from build123d import *

# Parameters (mm, degrees)
SKETCH1_R               = 2.5
BOSS_EXTRUDE1_DEPTH     = 7.5
BOSS_EXTRUDE2_DEPTH     = 20
BOSS_EXTRUDE3_DEPTH     = 7
CUT_EXTRUDE_THIN1_DEPTH = 7
SKETCH5_W               = 5.5
SKETCH5_H               = 11
CUT_EXTRUDE2_DEPTH      = 4
SKETCH6_W               = 5.5
SKETCH6_H               = 11
CUT_EXTRUDE3_DEPTH      = 4


with BuildPart() as part:
    # Sketch1 → Boss-Extrude1 (new body)
    with BuildSketch(Plane(origin=(0, 0, 0), x_dir=(1, 0, 0), z_dir=(0, 1, 0))):
        with BuildLine():
            Line((33, 16.75), (42.918528102, 1.646786754))
            ThreePointArc((42.918528102, 1.646786754), (43.410920998, 0), (42.918528102, -1.646786754))
            Line((42.918528102, -1.646786754), (33, -16.75))
            Line((33, -16.75), (33, -23.75))
            ThreePointArc((33, -23.75), (32.121320344, -25.871320344), (30, -26.75))
            Line((30, -26.75), (-30, -26.75))
            ThreePointArc((-30, -26.75), (-32.121320344, -25.871320344), (-33, -23.75))
            Line((-33, -23.75), (-33, -16.75))
            Line((-33, -16.75), (-42.918528102, -1.646786754))
            ThreePointArc((-42.918528102, -1.646786754), (-43.410920998, 0), (-42.918528102, 1.646786754))
            Line((-42.918528102, 1.646786754), (-33, 16.75))
            Line((-33, 16.75), (-33, 23.75))
            ThreePointArc((-33, 23.75), (-32.121320344, 25.871320344), (-30, 26.75))
            Line((-30, 26.75), (30, 26.75))
            ThreePointArc((30, 26.75), (32.121320344, 25.871320344), (33, 23.75))
            Line((33, 23.75), (33, 16.75))
        make_face()
        with Locations((38.5, 0)):
            Circle(SKETCH1_R, mode=Mode.SUBTRACT)
        with Locations((-38.5, 0)):
            Circle(SKETCH1_R, mode=Mode.SUBTRACT)
    extrude(amount=BOSS_EXTRUDE1_DEPTH)

    # Sketch2 → Boss-Extrude2 (add)
    with BuildSketch(Plane(origin=(0, 7.5, 0), x_dir=(1, 0, 0), z_dir=(0, 1, 0))):
        with BuildLine():
            Line((-30, 18.5), (30, 18.5))
            ThreePointArc((30, 18.5), (32.121320344, 17.621320344), (33, 15.5))
            Line((33, 15.5), (33, -15.5))
            ThreePointArc((33, -15.5), (32.121320344, -17.621320344), (30, -18.5))
            Line((30, -18.5), (-30, -18.5))
            ThreePointArc((-30, -18.5), (-32.121320344, -17.621320344), (-33, -15.5))
            Line((-33, -15.5), (-33, 15.5))
            ThreePointArc((-33, 15.5), (-32.121320344, 17.621320344), (-30, 18.5))
        make_face()
    extrude(amount=BOSS_EXTRUDE2_DEPTH)

    # Sketch3 → Boss-Extrude3 (add)
    with BuildSketch(Plane(origin=(0, 27.5, 0), x_dir=(1, 0, 0), z_dir=(0, 1, 0))):
        Polygon((-28, 13.5), (-22.4116483, 13.5), (-22.4116483, 6.5), (-23.4116483, 6.5), (-23.4116483, 10), (-27, 10), (-27, 6.5), (-28, 6.5), align=None)
        Polygon((-12, 13.5), (-6.4116483, 13.5), (-6.4116483, 6.5), (-7.4116483, 6.5), (-7.4116483, 10), (-11, 10), (-11, 6.5), (-12, 6.5), align=None)
        Polygon((4, 13.5), (9.5883517, 13.5), (9.5883517, 6.5), (8.5883517, 6.5), (8.5883517, 10), (5, 10), (5, 6.5), (4, 6.5), align=None)
        Polygon((20, 13.5), (25.5883517, 13.5), (25.5883517, 6.5), (24.5883517, 6.5), (24.5883517, 10), (21, 10), (21, 6.5), (20, 6.5), align=None)
        Polygon((-12, -6.5), (-11, -6.5), (-11, -10), (-7.4116483, -10), (-7.4116483, -6.5), (-6.4116483, -6.5), (-6.4116483, -13.5), (-12, -13.5), align=None)
        Polygon((4, -6.5), (5, -6.5), (5, -10), (8.5883517, -10), (8.5883517, -6.5), (9.5883517, -6.5), (9.5883517, -13.5), (4, -13.5), align=None)
        Polygon((20, -6.5), (21, -6.5), (21, -10), (24.5883517, -10), (24.5883517, -6.5), (25.5883517, -6.5), (25.5883517, -13.5), (20, -13.5), align=None)
        Polygon((-28, -6.5), (-27, -6.5), (-27, -10), (-23.4116483, -10), (-23.4116483, -6.5), (-22.4116483, -6.5), (-22.4116483, -13.5), (-28, -13.5), align=None)
    extrude(amount=BOSS_EXTRUDE3_DEPTH)

    # Sketch4 → Cut-Extrude-Thin1 (cut)
    with BuildSketch(Plane(origin=(0, 27.5, 0), x_dir=(1, 0, 0), z_dir=(0, 1, 0))):
        with BuildLine():
            Line((-28, 19.5), (28, 19.5))
            ThreePointArc((28, 19.5), (32.242640687, 17.742640687), (34, 13.5))
            Line((34, 13.5), (34, -13.5))
            ThreePointArc((34, -13.5), (32.242640687, -17.742640687), (28, -19.5))
            Line((28, -19.5), (-28, -19.5))
            ThreePointArc((-28, -19.5), (-32.242640687, -17.742640687), (-34, -13.5))
            Line((-34, -13.5), (-34, 13.5))
            ThreePointArc((-34, 13.5), (-32.242640687, 17.742640687), (-28, 19.5))
        make_face()
        with BuildLine():
            Line((-28, 16.5), (28, 16.5))
            ThreePointArc((28, 16.5), (30.121320344, 15.621320344), (31, 13.5))
            Line((31, 13.5), (31, -13.5))
            ThreePointArc((31, -13.5), (30.121320344, -15.621320344), (28, -16.5))
            Line((28, -16.5), (-28, -16.5))
            ThreePointArc((-28, -16.5), (-30.121320344, -15.621320344), (-31, -13.5))
            Line((-31, -13.5), (-31, 13.5))
            ThreePointArc((-31, 13.5), (-30.121320344, 15.621320344), (-28, 16.5))
        make_face(mode=Mode.SUBTRACT)
    extrude(amount=-CUT_EXTRUDE_THIN1_DEPTH, mode=Mode.SUBTRACT)

    # Sketch5 → Cut-Extrude2 (cut)
    with BuildSketch(Plane.XY.offset(18.5)):
        with Locations((-25.25, 13.1)):
            Rectangle(SKETCH5_W, SKETCH5_H)
        with Locations((-9.25, 13.1)):
            Rectangle(SKETCH5_W, SKETCH5_H)
        with Locations((6.75, 13.1)):
            Rectangle(SKETCH5_W, SKETCH5_H)
        with Locations((22.75, 13.1)):
            Rectangle(SKETCH5_W, SKETCH5_H)
    extrude(amount=-CUT_EXTRUDE2_DEPTH, mode=Mode.SUBTRACT)

    # Sketch6 → Cut-Extrude3 (cut)
    with BuildSketch(Plane(origin=(0, 0, -18.5), x_dir=(-1, 0, 0), z_dir=(0, 0, -1))):
        with Locations((-23.25, 13)):
            Rectangle(SKETCH6_W, SKETCH6_H)
        with Locations((-7.25, 13)):
            Rectangle(SKETCH6_W, SKETCH6_H)
        with Locations((8.75, 13)):
            Rectangle(SKETCH6_W, SKETCH6_H)
        with Locations((24.75, 13)):
            Rectangle(SKETCH6_W, SKETCH6_H)
    extrude(amount=-CUT_EXTRUDE3_DEPTH, mode=Mode.SUBTRACT)


solid = part.part
The listing builds one solid part. Answer for the finished solid, in the listing's coordinates (mm). A direction names the side the tool comes from. Give positions to 0.01 mm unless a question says otherwise; leave off trailing zeros. Loops run counter-clockwise (first coordinate to the right, second up) from the corner with the lowest first, then second, coordinate; pieces in that order, holes last.
Item 1: A cutting plane is placed at C-C (x = 11). Give the vertices of the cut face in (y, z).
Derived:
outline: (0, -26.75) - (7.5, -26.75) - (7.5, -18.5) - (20.5, -18.5) - (20.5, -16.5) - (27.5, -16.5) - (27.5, 16.5) - (20.5, 16.5) - (20.5, 18.5) - (7.5, 18.5) - (7.5, 26.75) - (0, 26.75) - close
Item 2: A cutting plane is placed at A-A (z = 0). Give the vertices of the cut face in (x, y), then the cut area to 3 significant figures.
Derived:
outline: (-43.41, 0) - (-41, 0) - (-41, 7.5) - (-43.41, 7.5) - close; (-36, 0) - (36, 0) - (36, 7.5) - (33, 7.5) - (33, 20.5) - (31, 20.5) - (31, 27.5) - (-31, 27.5) - (-31, 20.5) - (-33, 20.5) - (-33, 7.5) - (-36, 7.5) - close; (41, 0) - (43.41, 0) - (43.41, 7.5) - (41, 7.5) - close
area: 1,870 mm2
Item 3: A cutting plane is placed at D-D (z = -12). Give the vertices of the cut face in (x, y), then the cut area to 3 significant figures.
Derived:
outline: (-36.12, 0) - (36.12, 0) - (36.12, 7.5) - (33, 7.5) - (33, 20.5) - (31, 20.5) - (31, 27.5) - (25.59, 27.5) - (25.59, 34.5) - (20, 34.5) - (20, 27.5) - (9.59, 27.5) - (9.59, 34.5) - (4, 34.5) - (4, 27.5) - (-6.41, 27.5) - (-6.41, 34.5) - (-12, 34.5) - (-12, 27.5) - (-22.41, 27.5) - (-22.41, 34.5) - (-28, 34.5) - (-28, 27.5) - (-31, 27.5) - (-31, 20.5) - (-33, 20.5) - (-33, 7.5) - (-36.12, 7.5) - close
area: 1,990 mm2
Item 4: A cutting plane is placed at B-B (x = -37). Give the vertices of the cut face in (y, z).
Derived:
outline: (0, -10.66) - (7.5, -10.66) - (7.5, -2) - (0, -2) - close; (0, 2) - (7.5, 2) - (7.5, 10.66) - (0, 10.66) - close
Item 5: Each of these flat-tipped pins is pushed along its axis until it touches: pin 1 Ø4 at (x, y) = (-26, 31) entering from -Z; pin 2 Ø1.2 at (y, z) = (12.5, 17) entering from +X; pin 3 Ø4 at (x, z) = (-32.5, -5.5) entering from +Y. Where does it stop, or does it pass through?
Derived:
pin 1: stops at z = -13.5
pin 2: stops at x = 32.86
pin 3: stops at y = 27.5
Item 6: A tool of negligible diameter and unlimited length cuts with its end or side. For faces 1 (the flat face through (0, 24, -16.5)), 2 (the cylindrical face through (32.14, 13.91, 17.6)), 3 (the flat face through (10, 13, -17)), 4 (the flat face through (7, 7.6, 17)), 5 (the flat face through (21, 31, -8)), from which of +Z, -Z, +X, -X, +Y, -Y can it reach the whole face along a straight path? Write none if from no direction.
Derived:
face 1: -Z, +X, -X, +Y
face 2: +Z, +X, +Y
face 3: -Z
face 4: +Z
face 5: +Y
Item 7: Find the intervals of material crossed by line 1 along X through (y, z) = (5, 0); line 2 along X through (y, z) = (12, -13); line 3 along Z through (x, y) = (-4, 21), in increasing order.
Derived:
line 1: x = -43.41 to -41, -36 to 36, 41 to 43.41
line 2: x = -33 to 33
line 3: z = -16.5 to 16.5
Item 8: Determine the mould class of faces 6 (the flat face through (23, 18.5, -17)), 7 (the flat face through (-25, 31, -13.5)), 8 (the flat face through (25.588, 31, -10)) for opening direction X: +X half, -X half, draft (parallel to the pull), parting line (faces both ways), or undercut.
Derived:
face 6: undercut
face 7: draft
face 8: +X half
